Source: CAD feature listing. Evaluate the final solid. Frame: model axes, mm. Give positions to 0.01 mm unless a question says otherwise; leave off trailing zeros. Loops run counter-clockwise (first coordinate to the right, second up) from the corner with the lowest first, then second, coordinate; pieces in that order, holes last.
```python
from build123d import *

# Parameters (mm, degrees)
SKETCH1_R           = 40.5
SKETCH1_R_2         = 38.5
SKETCH1_R_3         = 19
BOSS_EXTRUDE1_DEPTH = 2
SKETCH1_3_R         = 40.5
SKETCH1_3_R_2       = 38.5
BOSS_EXTRUDE2_DEPTH = 8
FILLET1_R           = 1
FILLET2_R           = 1


with BuildPart() as part:
    # Sketch1 → Boss-Extrude1 (new body)
    with BuildSketch(Plane(origin=(0, 0, 0), x_dir=(1, 0, 0), z_dir=(0, 1, 0))):
        with Locations(Location((0, 0, 0), (0, 0, 270))):
            Circle(SKETCH1_R)
        Circle(SKETCH1_R_2, mode=Mode.SUBTRACT)
        Circle(SKETCH1_R_2)
        with Locations(Location((0, 0, 0), (0, 0, 270))):
            Circle(SKETCH1_R_3, mode=Mode.SUBTRACT)
    extrude(amount=BOSS_EXTRUDE1_DEPTH)

    # Sketch1_3 → Boss-Extrude2 (add)
    with BuildSketch(Plane(origin=(0, 0, 0), x_dir=(1, 0, 0), z_dir=(0, 1, 0))):
        with Locations(Location((0, 0, 0), (0, 0, 270))):
            Circle(SKETCH1_3_R)
        with Locations(Location((0, 0, 0), (0, 0, 270))):
            Circle(SKETCH1_3_R_2, mode=Mode.SUBTRACT)
    extrude(amount=BOSS_EXTRUDE2_DEPTH)

    # Fillet1
    fillet1_edges = [part.edges().sort_by_distance(p)[0] for p in [
        (0, 0, -40.5),
    ]]
    fillet(fillet1_edges, radius=FILLET1_R)

    # Fillet2
    fillet2_edges = [part.edges().sort_by_distance(p)[0] for p in [
        (0, 2, -38.5),
    ]]
    fillet(fillet2_edges, radius=FILLET2_R)


solid = part.part
```
(1) Ray query, line 1 along X through (y, z) = (6.1, 0); line 2 along Z through (x, y) = (-1, 5); line 3 along Y through (x, z) = (-19.5, -3.5). Return the intervals inside material, ascending.
A:
line 1: x = -40.5 to -38.5, 38.5 to 40.5
line 2: z = -40.49 to -38.49, 38.49 to 40.49
line 3: y = 0 to 2
(2) Section A-A, the plane x = 0. Return the cut outline in (y, z), then the cut area to 3 significant figures.
A:
outline: (0, -39.5) arc R1 ccw to (1, -40.5) - (8, -40.5) - (8, -38.5) - (3, -38.5) arc R1 cw to (2, -37.5) - (2, -19) - (0, -19) - close; (0, 19) - (2, 19) - (2, 37.5) arc R1 cw to (3, 38.5) - (8, 38.5) - (8, 40.5) - (1, 40.5) arc R1 ccw to (0, 39.5) - close
area: 110 mm2
(3) Section C-C, the plane y = 5.5. Return the cut outline in (x, z).
A:
outline: circle Ø81 at (0, 0); hole circle Ø77 at (0, 0)
(4) First-contact query: pin 1 (3 mm diameter, centred on x = -19, y = 7, fed in from -Z); pin 2 (6 mm diameter, centred on x = 26, z = 24.5, fed in from -Y); pin 3 (2 mm diameter, centred on x = 4.5, y = 4.5, fed in from +Z); pin 4 (4 mm diameter, centred on x = -2.5, y = 2, fed in from -Z). Flat tips, straight axial feed; report the tip coordinate or a pass-through.
A:
pin 1: stops at z = -36.52
pin 2: stops at y = 0
pin 3: stops at z = 40.35
pin 4: stops at z = -40.5
(5) Mould query, pull axis X, two halves, no side actions, for faces 1 (the flat face through (9, 2, -17)), 2 (the cylindrical face through (-37.584, 5.465, -8.346)), 3 (the flat face through (9, 0, 17)), 4 (the cylindrical face through (34.15, 4.45, 21.77)). Classes: pulls with the +X half, pulls with the -X half, needs draft (parallel to the pull), parting line crosses it, or undercut.
A:
face 1: undercut
face 2: undercut
face 3: needs draft
face 4: parting line crosses it
(6) Section B-B, the plane z = 0. Return the cut outline in (x, y).
A:
outline: (-40.5, 1) arc R1 ccw to (-39.5, 0) - (-19, 0) - (-19, 2) - (-37.5, 2) arc R1 cw to (-38.5, 3) - (-38.5, 8) - (-40.5, 8) - close; (19, 0) - (39.5, 0) arc R1 ccw to (40.5, 1) - (40.5, 8) - (38.5, 8) - (38.5, 3) arc R1 cw to (37.5, 2) - (19, 2) - close
